```python
from build123d import *

# Parameters (mm, degrees)
SKETCH1_W           = 133.5
SKETCH1_H           = 45
SKETCH1_R           = 3.05
SKETCH1_R_2         = 3.1
SKETCH1_W_2         = 5
SKETCH1_H_2         = 10
BOSS_EXTRUDE1_DEPTH = 5
FILLET1_R           = 1


with BuildPart() as part:
    # Sketch1 → Boss-Extrude1 (new body)
    with BuildSketch(Plane.XY):
        Rectangle(SKETCH1_W, SKETCH1_H)
        with Locations((25, 2.5)):
            Circle(SKETCH1_R, mode=Mode.SUBTRACT)
        with Locations(Location((-25, 2.5, 0), (0, 0, 180))):
            Circle(SKETCH1_R, mode=Mode.SUBTRACT)
        with Locations((-59.75, 0)):
            Circle(SKETCH1_R_2, mode=Mode.SUBTRACT)
        with Locations(Location((59.75, 0, 0), (0, 0, 180))):
            Circle(SKETCH1_R_2, mode=Mode.SUBTRACT)
        with Locations((-59.75, -12.5)):
            Rectangle(SKETCH1_W_2, SKETCH1_H_2, mode=Mode.SUBTRACT)
        with Locations((59.75, -12.5)):
            Rectangle(SKETCH1_W_2, SKETCH1_H_2, mode=Mode.SUBTRACT)
        with Locations((-59.75, 12.5)):
            Rectangle(SKETCH1_W_2, SKETCH1_H_2, mode=Mode.SUBTRACT)
        with Locations((59.75, 12.5)):
            Rectangle(SKETCH1_W_2, SKETCH1_H_2, mode=Mode.SUBTRACT)
    extrude(amount=BOSS_EXTRUDE1_DEPTH)

    # Fillet1
    fillet1_edges = [part.edges().sort_by_distance(p)[0] for p in [
        (66.75, -22.5, 2.5),
        (-66.75, -22.5, 2.5),
        (-66.75, 22.5, 2.5),
        (66.75, 22.5, 2.5),
    ]]
    fillet(fillet1_edges, radius=FILLET1_R)


solid = part.part
```
Input: part model. Units: mm. Frame: model coordinates. A direction names the side the tool comes from. Coordinates: 2 decimals unless noted, no trailing zeros. Loops run counter-clockwise (first coordinate to the right, second up) from the corner with the lowest first, then second, coordinate; pieces in that order, holes last. Notation, with made-up numbers: M -5.5,8.5 L 33.5,8.5 A23 cw 33.5,24.5 Z; hole C -24,64 d4. An arc over 180 degrees is marked long. Use a Markdown table: item, result. Add a question column.
1) Section C-C, the plane x = 25. Return the cut outline in (y, z), plus the area to 4 significant figures.
2) Line query: L1, parallel to X at y = 17, z = 3.7; L2, parallel to Y at x = -59.75, z = 3.15; L3, parallel to X at y = -2, z = 0.55. Output: solid intervals per line, ascending. Write a range as from..to.
3) Pin query (flat end, axial travel): P1, Ø6, axis at x = 9.5, y = -4.5, coming from the -Z side; P2, Ø5, axis at x = -59.75, y = 0, coming from the -Z side. Return the tip coordinate at first contact, or that it passes through.
4) Section B-B, the plane z = 4.25. Give the number of separate pieces and of enclosed holes in the cut face, plus the area to 3 significant figures.
5) Set-up query: faces 1 (the flat face through (62.25, 12, 2)), 2 (the flat face through (-1, 22.5, 2)). Return all of +Z, -Z, +X, -X, +Y, -Y with unobstructed straight access to the full face (end or side cutting, diameter ignored); none if empty.
6) Section A-A, the plane x = 59.75. Return the cut outline in (y, z).
7) Draft query along X for faces 3 (the flat face through (-66.75, 0, 2)), 4 (the flat face through (62.25, -13, 2)), 5 (the flat face through (66.75, 0, 2)). Return one class per face: +X half, -X half, draft (parallel to the pull), parting line (faces both ways), or undercut.
Answer below:
| question | item | result |
|---|---|---|
| 1 | outline | M -22.5,0 L -0.55,0 L -0.55,5 L -22.5,5 Z; M 5.55,0 L 22.5,0 L 22.5,5 L 5.55,5 Z |
| 1 | area | 194.5 mm2 |
| 2 | L1 | -66.75..-62.25, -57.25..57.25, 62.25..66.75 |
| 2 | L2 | -22.5..-17.5, -7.5..-3.1, 3.1..7.5, 17.5..22.5 |
| 2 | L3 | -66.75..-62.12, -57.38..57.38, 62.12..66.75 |
| 3 | P1 | z = 0 |
| 3 | P2 | through |
| 4 | separate pieces | 1 |
| 4 | enclosed holes | 8 |
| 4 | area | 5,690 mm2 |
| 5 | face 1 | +Z, -Z |
| 5 | face 2 | +Z, -Z, +X, -X, +Y |
| 6 | outline | M -22.5,0 L -17.5,0 L -17.5,5 L -22.5,5 Z; M -7.5,0 L -3.1,0 L -3.1,5 L -7.5,5 Z; M 3.1,0 L 7.5,0 L 7.5,5 L 3.1,5 Z; M 17.5,0 L 22.5,0 L 22.5,5 L 17.5,5 Z |
| 7 | face 3 | -X half |
| 7 | face 4 | undercut |
| 7 | face 5 | +X half |
